Verification items for the finished model (mm, model axes). A direction names the side the tool comes from. Coordinates: 2 decimals unless noted, no trailing zeros. Write each loop counter-clockwise with the first axis right and the second up, starting at its lowest first coordinate (ties: lowest second). Pieces come first, ordered by that corner, then holes. Notation, with made-up numbers: (21, 41) -> (36, 41) arc R30 cw to (36, 72) -> close; hole circle Ø10 at (54.25, 75.25). An arc over 180 degrees is marked (long way). Use a Markdown table: item, result. Add a question column.
Autodesk Inventor part; units mm, degrees
ref_plane "YZ Plane" through (0, 0, 0) normal (1, 0, 0) x (0, 1, 0)
ref_plane "XZ Plane" through (0, 0, 0) normal (0, 1, 0) x (-1, 0, 0)
ref_plane "XY Plane" through (0, 0, 0) normal (0, 0, 1) x (1, 0, 0)
sketch "Sketch1" plane through (0, 0, 0) normal (0, 1, 0) x (-1, 0, 0)
  line L0 (0, 0) -> (209, 0)
  line L1 (209, -23) -> (0, -23)
  line L2 (0, -23) -> (0, 0)
  line L3 (209, -6.5) -> (215, -6.5)
  line L4 (215, -6.5) -> (215, -16.5)
  line L5 (215, -16.5) -> (209, -16.5)
  line L6 (209, 0) -> (209, -6.5)
  line L7 (209, -16.5) -> (209, -23)
  dimension "d0" = 209
  dimension "d1" = 23
  dimension "d3" = 6
  dimension "d4" = 10
extrude "Extrusion1" add sketch "Sketch1" along normal blind 6
sketch "Sketch2" plane through (0, 6, 0) normal (0, 1, 0) x (1, 0, 0)
  line L0 (-209, 0) -> (0, 0)
  line L1 (-209, 0) -> (-198.55, 0)
  line L2 (-198.55, 0) -> (-188.1, 0)
  line L3 (-188.1, 0) -> (-188.1, -6)
  line L4 (-188.1, -6) -> (-198.55, -6)
  line L5 (-198.55, -6) -> (-198.55, 0)
  line L6 (-209, 23) -> (-209, 16.5)
  line L7 (0, 23) -> (-209, 23)
  line L8 (-198.55, 23) -> (-188.1, 23)
  line L9 (-188.1, 23) -> (-188.1, 29)
  line L10 (-188.1, 29) -> (-198.55, 29)
  line L11 (-198.55, 29) -> (-198.55, 23)
  dimension "d7" = 10.45
  dimension "d8" = 10.45
  dimension "d9" = 6
  dimension "d10" = 10.45
  dimension "d11" = 10.45
  dimension "d12" = 6
extrude "Extrusion2" add sketch "Sketch2" against normal blind 6
pattern_linear "Rectangular Pattern1" count 10 spacing 20.9 along (1, 0, 0) of "Extrusion2"
properties part number "g_arm 4"
1) Set-up check for faces 1 (the face through (-131, 3, 6)), 2 (the face through (-120, 3, -23)), 3 (the face through (-106, 0, -11)), 4 (the face through (-73.15, 3, 3)), 5 (the face through (-204, 3, 0)): record each of +Z, -Z, +X, -X, +Y, -Y from which the full face is reachable in a straight line by a thin tool's end or side.
2) Thickness scan on L1, parallel to X at y = 2.25, z = -4; L2, parallel to Z at x = -35.5, y = 5. Record the ranges inside material, lowest first.
3) Cross-section at A-A on x = -200.5. Record the boundary of the cut face in (y, z), then the cut area to 3 significant figures.
4) Gauge pin test, flat ends, axial feed: pin 1 (1.8 mm diameter, centred on x = -213, y = 2, fed in from +Z); pin 2 (1.8 mm diameter, centred on x = -182.5, y = 2.5, fed in from +Z); pin 3 (1.8 mm diameter, centred on y = 4, z = 4.5, fed in from -X). Record the tip position at first contact, or that the pin passes through.
Returned:
| question | item | result |
|---|---|---|
| 1 | face 1 | +Z, +X, -X, +Y, -Y |
| 1 | face 2 | -Z, +Y, -Y |
| 1 | face 3 | +Z, -Z, +X, -X, -Y |
| 1 | face 4 | +Z, +Y, -Y |
| 1 | face 5 | +Z, -X, +Y, -Y |
| 2 | L1 | x = -209 to 0 |
| 2 | L2 | z = -23 to 0 |
| 3 | outline | (0, -23) -> (6, -23) -> (6, 0) -> (0, 0) -> close |
| 3 | area | 138 mm² |
| 4 | pin 1 | stops at z = -6.5 |
| 4 | pin 2 | stops at z = 0 |
| 4 | pin 3 | stops at x = -198.55 |
